Can you work these out from the model? Positions are in its coordinate system, mm. A direction names the side the tool comes from. Coordinates: 2 decimals unless noted, no trailing zeros. Order: outer loops, then holes, each group sorted by start corner. A loop starts at its lowest first (then second) coordinate and runs counter-clockwise, first axis right, second up. Notation, with made-up numbers: (84, 36.5) - (134, 36.5) arc R20 ccw to (134, 44.5) - close; hole circle Ø10 at (-28, 45). An arc over 180 degrees is marked (long way). Return JSON: item names as keys, results as strings. Group by question number.
1) If we mould it in two halves opening along Y, with no side actions, what happens to faces 1 (the face through (-0.54, -2.44, 6.59)), 2 (the face through (-2, 2, 13)), 3 (the face through (6.633, -6.083, 12.493))? For each: pulls with the +Y half, pulls with the -Y half, needs draft (parallel to the pull), parting line crosses it, or undercut.
2) Imagine slicing it at A-A (x = 0). Write out the boundary of the cut face in (y, z), and give its area (3 significant figures).
3) Imagine slicing it at C-C (y = -3.25). Write out the boundary of the cut face in (x, z).
4) Imagine slicing it at D-D (z = 6). Write out the boundary of the cut face in (x, y), and give its area (3 significant figures).
5) For pin 1 Ø5 at (y, z) = (-2, 6.5) entering from -X; pin 2 Ø3 at (y, z) = (-3, 10) entering from +X; pin 3 Ø4 at (x, z) = (6.5, 10.5) entering from -Y, each with a flat end and sliding along its axis, tell me the tip position at first contact or that it passes through.
6) Which directions (+Z, -Z, +X, -X, +Y, -Y) give clear straight access to the entire face, cutting with the end or side of a thin tool? Please do faces 4 (the face through (-2, 2, 0)), 5 (the face through (-2, 6, 12)).
7) If I drill on line 1 along Z through (x, y) = (4.5, 7); line 2 along Y through (x, z) = (0, 7); line 3 along X through (y, z) = (-1, 4.25), over which ranges is the centre line in solid material (lowest first)?
```python
from build123d import *

# Parameters (mm, degrees)
SKETCH_1_R          = 9
EXTRUDE_1_DEPTH     = 13
CUT_EXTRUDE_START   = -12
SKETCH_2_R          = 9
SKETCH_2_R_2        = 6
CUT_EXTRUDE_1_DEPTH = 11
SKETCH_3_R          = 2.5
CUT_EXTRUDE_2_DEPTH = 19.193405399


with BuildPart() as part:
    # 草图1 → 凸台-拉伸1 (new body)
    with BuildSketch(Plane.XY):
        with Locations(Location((0, 0, 0), (0, 0, 180))):
            Circle(SKETCH_1_R)
    extrude(amount=EXTRUDE_1_DEPTH)

    # 草图2 → 切除-拉伸1 (cut)
    with BuildSketch(Plane.XY.offset(13).offset(CUT_EXTRUDE_START)):
        with Locations(Location((0, 0, 0), (0, 0, 180))):
            Circle(SKETCH_2_R)
        Circle(SKETCH_2_R_2, mode=Mode.SUBTRACT)
    extrude(amount=CUT_EXTRUDE_1_DEPTH, mode=Mode.SUBTRACT)

    # 草图3 → 切除-拉伸2 (cut, through all)
    with BuildSketch(Plane.XY.offset(13)):
        Circle(SKETCH_3_R)
    extrude(amount=-CUT_EXTRUDE_2_DEPTH, mode=Mode.SUBTRACT)


solid = part.part
```
Calculated:
{
 "1": {"face 1": "undercut", "face 2": "needs draft", "face 3": "parting line crosses it"},
 "2": {"outline": "(-9, 0) - (-2.5, 0) - (-2.5, 13) - (-9, 13) - (-9, 12) - (-6, 12) - (-6, 1) - (-9, 1) - close; (2.5, 0) - (9, 0) - (9, 1) - (6, 1) - (6, 12) - (9, 12) - (9, 13) - (2.5, 13) - close", "area": "103 mm2"},
 "3": {"outline": "(-8.39, 0) - (8.39, 0) - (8.39, 1) - (5.04, 1) - (5.04, 12) - (8.39, 12) - (8.39, 13) - (-8.39, 13) - (-8.39, 12) - (-5.04, 12) - (-5.04, 1) - (-8.39, 1) - close"},
 "4": {"outline": "circle Ø12 at (0, 0); hole circle Ø5 at (0, 0)", "area": "93.5 mm2"},
 "5": {"pin 1": "x = -6", "pin 2": "x = 5.81", "pin 3": "y = -7.36"},
 "6": {"face 4": "-Z, +X, -X, +Y, -Y", "face 5": "none"},
 "7": {"line 1": "0 to 1, 12 to 13", "line 2": "-6 to -2.5, 2.5 to 6", "line 3": "-5.92 to -2.29, 2.29 to 5.92"}
}
